Autodesk Inventor part; units mm, degrees
ref_plane "YZ Plane" through (0, 0, 0) normal (1, 0, 0) x (0, 1, 0)
ref_plane "XZ Plane" through (0, 0, 0) normal (0, 1, 0) x (-1, 0, 0)
ref_plane "XY Plane" through (0, 0, 0) normal (0, 0, 1) x (1, 0, 0)
sketch "Sketch1" plane through (0, 0, 0) normal (0, 0, 1) x (1, 0, 0)
  line L0 (0, 0) -> (38.1, 0)
  line L1 (38.1, 0) -> (38.1, -85.725)
  line L2 (38.1, -85.725) -> (0, -85.725)
  line L3 (0, -85.725) -> (0, 0)
  line L4 (38.1, -85.725) -> (38.1, -123.825)
  line L5 (38.1, -123.825) -> (0, -85.725)
  dimension "d0" = 38.1
  dimension "d1" = 85.725
  dimension "d4" = 38.1
extrude "Extrusion1" add sketch "Sketch1" along normal blind 2.3622 contours L0 L1 L2 L3
extrude "Extrusion2" add sketch "Sketch1" along normal blind 2.3622 contours L2 L4 L5
sketch "Sketch2" plane through (0, 0, 2.3622) normal (0, 0, 1) x (1, 0, 0)
  line L0 (0, -85.725) -> (38.1, -123.825)
  line L1 (38.1, -123.825) -> (38.1, 0)
  line L2 (38.1, -115.4195) -> (4.2028, -81.5222)
  line L3 (0, -85.725) -> (4.2028, -81.5222)
  line L4 (38.1, -115.4195) -> (38.1, -123.825)
  line L5 (38.1, -123.825) -> (0, -85.725)
  line L6 (0, -85.725) -> (4.2028, -81.5222)
  line L7 (4.2028, -81.5222) -> (38.1, -115.4195)
  line L8 (38.1, -115.4195) -> (38.1, -123.825)
  line L9 (38.1, -123.825) -> (0, -85.725)
  dimension "d7" = 5.9436
extrude "Extrusion3" cut sketch "Sketch2" against normal blind 25.4
sketch "Sketch3" plane through (0, 0, 0) normal (0, 0, -1) x (-1, 0, 0)
  circle A0 centre (-25.4, -15.24) radius 1.4986
  circle A1 centre (-25.4, -76.2) radius 1.4986
  line L0 (0, 0) -> (-38.1, 0)
  line L1 (-38.1, 0) -> (-38.1, -115.4195)
  dimension "d19" = 2.9972
  dimension "d20" = 2.9972
  dimension "d21" = 15.24
  dimension "d22" = 12.7
  dimension "d23" = 12.7
extrude "Extrusion4" cut sketch "Sketch3" against normal blind 25.4
properties part number "Plate_InnerSide_Poly" material "Polycarbonate, Clear"
Can you work these out from the model? Positions are in its coordinate system, mm. Coordinates: 2 decimals unless noted, no trailing zeros. Loops run counter-clockwise (first coordinate to the right, second up) from the corner with the lowest first, then second, coordinate; pieces in that order, holes last. Notation, with made-up numbers: (-32, 45.25) - (-27, 45.25) arc R21 ccw to (-27, 62.25) - close; hole circle Ø1 at (-7, -17). An arc over 180 degrees is marked (long way). Put each result on its own line as item: value. Start each with the question number.
Item 1: Suppose I cut it at A-A (z = 1.7). Please give me the cut outline in (x, y) (1 decimal), and give its area (3 significant figures).
Item 2: If we mould it in two halves opening along X, with no side actions, what happens to faces 1 (the face through (0, -43, 1)), 2 (the face through (19, 0, 1)), 3 (the face through (2.072, -83.653, 1.198))? For each: +X half, -X half, draft (parallel to the pull), parting line (faces both ways), or undercut.
Item 3: Suppose I cut it at B-B (y = -76.2). Please give me the cut outline in (x, z), and give its area (3 significant figures).
Item 4: Suppose I cut it at C-C (x = 25.4). Please give me the cut outline in (y, z).
Item 5: Suppose I cut it at D-D (x = 12). Please give me the cut outline in (y, z).
Item 6: If I drill on line 1 along X through (y, z) = (-76.2, 1.4); line 2 along Y through (x, z) = (26, 2); line 3 along Y through (x, z) = (25.4, 1.85), over which ranges is the centre line in solid material (lowest first)?
Here are the results:
1. outline: (0, -85.7) - (4.2, -81.5) - (38.1, -115.4) - (38.1, 0) - (0, 0) - close; hole circle Ø3 at (25.4, -76.2); hole circle Ø3 at (25.4, -15.2)
1. area: 3,680 mm²
2. face 1: -X half
2. face 2: draft
2. face 3: undercut
3. outline: (0, 0) - (23.9, 0) - (23.9, 2.36) - (0, 2.36) - close; (26.9, 0) - (38.1, 0) - (38.1, 2.36) - (26.9, 2.36) - close
3. area: 82.9 mm²
4. outline: (-102.72, 0) - (-77.7, 0) - (-77.7, 2.36) - (-102.72, 2.36) - close; (-74.7, 0) - (-16.74, 0) - (-16.74, 2.36) - (-74.7, 2.36) - close; (-13.74, 0) - (0, 0) - (0, 2.36) - (-13.74, 2.36) - close
5. outline: (-89.32, 0) - (0, 0) - (0, 2.36) - (-89.32, 2.36) - close
6. line 1: 0 to 23.9, 26.9 to 38.1
6. line 2: -103.32 to -77.57, -74.83 to -16.61, -13.87 to 0
6. line 3: -102.72 to -77.7, -74.7 to -16.74, -13.74 to 0
